Geometry check sheet. Reference: the model listing, model coordinates, mm. A direction names the side the tool comes from. Give positions to 0.01 mm unless a question says otherwise; leave off trailing zeros. Loops run counter-clockwise (first coordinate to the right, second up) from the corner with the lowest first, then second, coordinate; pieces in that order, holes last.
1. Cross-section at C-C, the plane z = -4. Record the cut outline in (x, y), plus the area to 3 significant figures.
2. Material ranges on L1, parallel to X at y = 10, z = 0 (3 decimals); L2, parallel to Z at x = -25.4, y = 6 (3 decimals); L3, parallel to Z at x = -7, y = 25, recorded low to high.
3. Release check for a two-part mould opening along Z. For faces 4 (the flat face through (-27, 0, 3)), 5 (the cylindrical face through (-22.37, 6.26, 0.95)), 6 (the cylindrical face through (-6.261, 19.056, 0.279)) record: +Z half, -Z half, draft (parallel to the pull), parting line (faces both ways), or undercut.
4. Tool access check on faces 1 (the cylindrical face through (-6.26, 28.43, 0.95)), 2 (the cylindrical face through (-19.343, 6.261, 1.907)), 3 (the flat face through (0, 27, 3)). Record the directions out of +Z, -Z, +X, -X, +Y, -Y that give a thin tool (end or side, any length) a straight path to the whole face; none if there is none.
5. Cross-section at A-A, the plane z = 0. Record the cut outline in (x, y) (3 decimals).
6. Cross-section at B-B, the plane x = -4. Record the cut outline in (y, z) (3 decimals), plus the area to 3 significant figures.
7. Cross-section at D-D, the plane z = 2.25. Record the cut outline in (x, y), plus the area to 3 significant figures.
8. Go/stop test with flat-tipped pins: pin 1 Ø5 at (x, z) = (-25.4, 0) entering from +Y; pin 2 Ø2 at (x, y) = (-17, 22.5) entering from -Z; pin 3 Ø4 at (y, z) = (17.5, 2.5) entering from -X. Record where each tip stops, or that it passes through.
from build123d import *

# Parameters (mm, degrees)
F0_R        = 6.35
F0_R_2      = 3.175
F1_DEPTH    = 12.7
F2_R        = 6.35
F2_R_2      = 3.175
F3_DEPTH    = 12.7
F1_FACE_R   = 6.35
F1_FACE_R_2 = 3.175


with BuildPart() as f1:
    # F0 (on Right) → F1 (new body)
    with BuildSketch(Plane.YZ):
        with Locations((25.4, 0)):
            Circle(F0_R)
        with Locations((25.4, 0)):
            Circle(F0_R_2, mode=Mode.SUBTRACT)
    extrude(amount=-F1_DEPTH)



with BuildPart() as f3:
    # F2 (on Front) → F3 (new body)
    with BuildSketch(Plane.XZ):
        with Locations((-25.4, 0)):
            Circle(F2_R)
        with Locations((-25.4, 0)):
            Circle(F2_R_2, mode=Mode.SUBTRACT)
    extrude(amount=-F3_DEPTH)


with BuildPart() as f1_1:
    add(f1.part)

    add(f3.part)  # F5 merges F3
    # F5: sweep along a path in F4
    with BuildLine(Plane.XY) as f5_path:
        ThreePointArc((-12.7, 38.1), (-30.6605122421, 30.6605122421), (-38.1, 12.7))
    # F1_face (on face) → F5 (sweep)
    with BuildSketch(Plane(origin=(-12.7, 25.4, 0), x_dir=(0, 1, 0), z_dir=(-1, 0, 0))):
        Circle(F1_FACE_R)
        Circle(F1_FACE_R_2, mode=Mode.SUBTRACT)
    sweep(path=f5_path.line)


solid = f1_1.part
Result:
1. outline: (-30.33, 0) - (-20.47, 0) - (-20.47, 12.7) arc R7.77 cw to (-12.7, 20.47) - (0, 20.47) - (0, 30.33) - (-12.7, 30.33) arc R17.63 ccw to (-30.33, 12.7) - close
1. area: 447 mm2
2. L1: x = -31.75 to -28.575, -22.225 to -19.05
2. L2: z = -6.35 to -3.175, 3.175 to 6.35
2. L3: z = -6.34 to -3.15, 3.15 to 6.34
3. face 4: draft
3. face 5: undercut
3. face 6: parting line
4. face 1: +X
4. face 2: -Y
4. face 3: +Z, -Z, +X, +Y, -Y
5. outline: (-31.75, 0) - (-28.575, 0) - (-28.575, 12.7) arc R15.875 cw to (-12.7, 28.575) - (0, 28.575) - (0, 31.75) - (-12.7, 31.75) arc R19.05 ccw to (-31.75, 12.7) - close; (-22.225, 0) - (-19.05, 0) - (-19.05, 12.7) arc R6.35 cw to (-12.7, 19.05) - (0, 19.05) - (0, 22.225) - (-12.7, 22.225) arc R9.525 ccw to (-22.225, 12.7) - close
6. outline: circle Ø12.7 at (25.4, 0); hole circle Ø6.35 at (25.4, 0)
6. area: 95.0 mm2
7. outline: (-31.34, 0) - (-27.64, 0) - (-27.64, 12.7) arc R14.94 cw to (-12.7, 27.64) - (0, 27.64) - (0, 31.34) - (-12.7, 31.34) arc R18.64 ccw to (-31.34, 12.7) - close; (-23.16, 0) - (-19.46, 0) - (-19.46, 12.7) arc R6.76 cw to (-12.7, 19.46) - (0, 19.46) - (0, 23.16) - (-12.7, 23.16) arc R10.46 ccw to (-23.16, 12.7) - close
7. area: 335 mm2
8. pin 1: stops at y = 28.79
8. pin 2: stops at z = -6.27
8. pin 3: stops at x = -31.35
